Input: part model. Units: mm. Frame: model coordinates. A direction names the side the tool comes from. Coordinates: 2 decimals unless noted, no trailing zeros. Order: outer loops, then holes, each group sorted by start corner. A loop starts at its lowest first (then second) coordinate and runs counter-clockwise, first axis right, second up. Notation, with made-up numbers: (83.25, 18.25) - (92.25, 18.25) arc R26 ccw to (92.25, 48.25) - close; hole circle Ø3 at (46, -21). An arc over 180 degrees is marked (long way). Use a Markdown table: item, result. Add a question column.
from build123d import *

# Parameters (mm, degrees)
SKETCH1_W           = 100
SKETCH1_H           = 100
BOSS_EXTRUDE1_DEPTH = 100
SKETCH2_R           = 15
CUT_EXTRUDE2_DEPTH  = 10
SKETCH3_R           = 10
CUT_EXTRUDE3_DEPTH  = 10
CUT_EXTRUDE5_DEPTH  = 10
SKETCH11_R          = 12.5
CUT_EXTRUDE6_DEPTH  = 10
SKETCH12_R          = 12.5
CUT_EXTRUDE7_DEPTH  = 10
SKETCH13_R          = 12
CUT_EXTRUDE12_DEPTH = 10


with BuildPart() as part:
    # Sketch1 → Boss-Extrude1 (new body)
    with BuildSketch(Plane(origin=(0, 0, 0), x_dir=(1, 0, 0), z_dir=(0, 1, 0))):
        with Locations((9.059630809, -2.226900841)):
            Rectangle(SKETCH1_W, SKETCH1_H)
    extrude(amount=BOSS_EXTRUDE1_DEPTH)

    # Sketch2 → Cut-Extrude2 (cut)
    with BuildSketch(Plane.XZ):
        with Locations(Location((10.537704993, 2.705564775, 0), (0, 0, 270))):
            Circle(SKETCH2_R)
    extrude(amount=-CUT_EXTRUDE2_DEPTH, mode=Mode.SUBTRACT)

    # Sketch3 → Cut-Extrude3 (cut)
    with BuildSketch(Plane(origin=(59.059630809, 0, 0), x_dir=(0, 0, -1), z_dir=(1, 0, 0))):
        with Locations((-2.226900841, 50)):
            Circle(SKETCH3_R)
        with Locations((22.5218365, 25.251262658)):
            Circle(SKETCH3_R)
        with Locations((-26.975638183, 74.748737342)):
            Circle(SKETCH3_R)
    extrude(amount=-CUT_EXTRUDE3_DEPTH, mode=Mode.SUBTRACT)

    # Sketch5 → Cut-Extrude5 (cut)
    with BuildSketch(Plane(origin=(0, 0, -47.773099159), x_dir=(-1, 0, 0), z_dir=(0, 0, -1))):
        with BuildLine():
            ThreePointArc((-34.059630809, 62.5), (-25.220796045, 66.161165235), (-21.559630809, 75))
            Line((-21.559630809, 75), (-34.059630809, 75))
            Line((-34.059630809, 75), (-34.059630809, 62.5))
        make_face()
        with BuildLine():
            Line((-34.059630809, 75), (-21.559630809, 75))
            ThreePointArc((-21.559630809, 75), (-42.898465574, 83.838834765), (-34.059630809, 62.5))
            Line((-34.059630809, 62.5), (-34.059630809, 75))
        make_face()
        with BuildLine():
            ThreePointArc((28.440369191, 75), (15.940369191, 87.5), (3.440369191, 75))
            Line((3.440369191, 75), (15.940369191, 75))
            Line((15.940369191, 75), (15.940369191, 62.5))
            ThreePointArc((15.940369191, 62.5), (24.779203955, 66.161165235), (28.440369191, 75))
        make_face()
        with BuildLine():
            Line((15.940369191, 75), (3.440369191, 75))
            ThreePointArc((3.440369191, 75), (7.101534426, 66.161165235), (15.940369191, 62.5))
            Line((15.940369191, 62.5), (15.940369191, 75))
        make_face()
        with BuildLine():
            ThreePointArc((-21.559630809, 25), (-25.220796045, 33.838834765), (-34.059630809, 37.5))
            Line((-34.059630809, 37.5), (-34.059630809, 25))
            Line((-34.059630809, 25), (-21.559630809, 25))
        make_face()
        with BuildLine():
            Line((-34.059630809, 25), (-34.059630809, 37.5))
            ThreePointArc((-34.059630809, 37.5), (-42.898465574, 16.161165235), (-21.559630809, 25))
            Line((-21.559630809, 25), (-34.059630809, 25))
        make_face()
        with BuildLine():
            ThreePointArc((28.440369191, 25), (24.779203955, 33.838834765), (15.940369191, 37.5))
            Line((15.940369191, 37.5), (15.940369191, 25))
            Line((15.940369191, 25), (3.440369191, 25))
            ThreePointArc((3.440369191, 25), (15.940369191, 12.5), (28.440369191, 25))
        make_face()
        with BuildLine():
            Line((15.940369191, 25), (15.940369191, 37.5))
            ThreePointArc((15.940369191, 37.5), (7.101534426, 33.838834765), (3.440369191, 25))
            Line((3.440369191, 25), (15.940369191, 25))
        make_face()
    extrude(amount=-CUT_EXTRUDE5_DEPTH, mode=Mode.SUBTRACT)

    # Sketch11 → Cut-Extrude6 (cut)
    with BuildSketch(Plane(origin=(0, 100, 0), x_dir=(1, 0, 0), z_dir=(0, 1, 0))):
        with Locations(Location((34.059630809, -27.226900841, 0), (0, 0, 270))):
            Circle(SKETCH11_R)
        with Locations(Location((34.059630809, 22.773099159, 0), (0, 0, 270))):
            Circle(SKETCH11_R)
        with Locations(Location((9.059630809, -2.226900841, 0), (0, 0, 270))):
            Circle(SKETCH11_R)
        with Locations(Location((-15.940369191, 22.773099159, 0), (0, 0, 270))):
            Circle(SKETCH11_R)
        with Locations(Location((-15.940369191, -27.226900841, 0), (0, 0, 270))):
            Circle(SKETCH11_R)
    extrude(amount=-CUT_EXTRUDE6_DEPTH, mode=Mode.SUBTRACT)

    # Sketch12 → Cut-Extrude7 (cut)
    with BuildSketch(Plane.XY.offset(52.226900841)):
        with Locations((9.059630809, 78.388490916)):
            Circle(SKETCH12_R)
        with Locations((9.059630809, 28.388490916)):
            Circle(SKETCH12_R)
    extrude(amount=-CUT_EXTRUDE7_DEPTH, mode=Mode.SUBTRACT)

    # Sketch13 → Cut-Extrude12 (cut)
    with BuildSketch(Plane.ZY.offset(40.940369191)):
        with Locations((-22.773099159, 25)):
            Circle(SKETCH13_R)
        with Locations((-22.773099159, 73.709409376)):
            Circle(SKETCH13_R)
        with Locations((2.226900841, 75)):
            Circle(SKETCH13_R)
        with Locations((2.226900841, 25)):
            Circle(SKETCH13_R)
        with Locations((27.226900841, 25)):
            Circle(SKETCH13_R)
        with Locations((27.226900841, 75)):
            Circle(SKETCH13_R)
    extrude(amount=-CUT_EXTRUDE12_DEPTH, mode=Mode.SUBTRACT)


solid = part.part
1) Contact query for flat-ended pins moving along their axis: P1, Ø4, axis at y = 22.5, z = -29, coming from the -X side; P2, Ø12.5, axis at x = 37, y = 23, coming from the -Z side; P3, Ø6, axis at y = 28, z = -21, coming from the +X side. Output: stop coordinate, or through.
2) Cut plane A-A (y = 50). Return the cut outline in (x, z).
3) Material intervals for L1, parallel to Z at x = -34, y = 24.5; L2, parallel to X at y = 95, z = -24; L3, parallel to X at y = 67, z = -41.5, sorted ascending.
4) Reachability of faces 1 (the flat face through (34, 90, -23)), 2 (the flat face through (11, 10, 3)), 3 (the flat face through (49.06, 25, -22)), 4 (the cylindrical face through (-36.01, 13.285, -0.374)), 5 (the cylindrical face through (7.43, 90.78, 47.3)) from +Z, -Z, +X, -X, +Y, -Y: full face, straight path, thin tool, end or side. Return the list, or none.
5) Cut plane C-C (y = 93). Return the cut outline in (x, z), and give its area (3 significant figures).
6) Cut plane B-B (z = 8.5). Return the cut outline in (x, y).
7) Cut plane D-D (x = 42.5). Return the cut outline in (y, z).
8) Pull-direction query (Z, two-part tool) for faces 6 (the flat face through (-16, 25, -37.773)), 7 (the flat face through (-3, 0, -10)), 8 (the cylindrical face through (54.13, 83.18, 21.6)), 9 (the flat face through (8, 49, 52.227)); classes: pulls with the +Z half, pulls with the -Z half, needs draft (parallel to the pull), parting line crosses it, or undercut.
Computed:
| question | item | result |
|---|---|---|
| 1 | P1 | stops at x = -30.94 |
| 1 | P2 | stops at z = -37.77 |
| 1 | P3 | stops at x = 49.06 |
| 2 | outline | (-40.94, -47.77) - (59.06, -47.77) - (59.06, -7.77) - (49.06, -7.77) - (49.06, 12.23) - (59.06, 12.23) - (59.06, 52.23) - (-40.94, 52.23) - close |
| 3 | L1 | z = -47.77 to -34.76, -10.78 to -9.76, 14.22 to 15.24, 39.22 to 52.23 |
| 3 | L2 | x = -40.94 to -28.38, -3.5 to 21.62, 46.5 to 59.06 |
| 3 | L3 | x = -40.94 to -25.55, -6.34 to 24.45, 43.66 to 59.06 |
| 4 | face 1 | +Y |
| 4 | face 2 | -Y |
| 4 | face 3 | +X |
| 4 | face 4 | -X |
| 4 | face 5 | +Z |
| 5 | outline | (-40.94, -47.77) - (59.06, -47.77) - (59.06, 52.23) - (-40.94, 52.23) - close; hole circle Ø25 at (-15.94, -22.77); hole circle Ø25 at (-15.94, 27.23); hole circle Ø25 at (9.06, 2.23); hole circle Ø25 at (34.06, -22.77); hole circle Ø25 at (34.06, 27.23) |
| 5 | area | 7,550 mm2 |
| 6 | outline | (-40.94, 0) - (-3.3, 0) - (-3.3, 10) - (24.37, 10) - (24.37, 0) - (59.06, 0) - (59.06, 42.21) - (49.06, 42.21) - (49.06, 57.79) - (59.06, 57.79) - (59.06, 100) - (19.87, 100) - (19.87, 90) - (-1.75, 90) - (-1.75, 100) - (-40.94, 100) - (-40.94, 85.23) - (-30.94, 85.23) - (-30.94, 64.77) - (-40.94, 64.77) - (-40.94, 35.23) - (-30.94, 35.23) - (-30.94, 14.77) - (-40.94, 14.77) - close |
| 7 | outline | (0, -47.77) - (15.78, -47.77) - (15.78, -37.77) - (34.22, -37.77) - (34.22, -47.77) - (65.78, -47.77) - (65.78, -37.77) - (84.22, -37.77) - (84.22, -47.77) - (100, -47.77) - (100, -31.99) - (90, -31.99) - (90, -13.55) - (100, -13.55) - (100, 18.01) - (90, 18.01) - (90, 36.45) - (100, 36.45) - (100, 52.23) - (0, 52.23) - close |
| 8 | face 6 | pulls with the -Z half |
| 8 | face 7 | needs draft |
| 8 | face 8 | undercut |
| 8 | face 9 | pulls with the +Z half |
